from build123d import *

# Parameters (mm, degrees)
SKIZZE1_W                       = 26
SKIZZE1_H                       = 15
AUFSATZ_LINEAR_AUSTRAGEN1_DEPTH = 5
SCHNITT_LINEAR_AUSTRAGEN1_DEPTH = 15
SKIZZE3_W                       = 10
SKIZZE3_H                       = 15
SCHNITT_LINEAR_AUSTRAGEN2_DEPTH = 1.55


with BuildPart() as part:
    # Skizze1 → Aufsatz-Linear austragen1 (new body)
    with BuildSketch(Plane.XY):
        with Locations((13, 7.5)):
            Rectangle(SKIZZE1_W, SKIZZE1_H)
    extrude(amount=AUFSATZ_LINEAR_AUSTRAGEN1_DEPTH)

    # Skizze2 → Schnitt-Linear austragen1 (cut)
    with BuildSketch(Plane.ZY):
        with BuildLine():
            Line((5, 9.247140521), (5, 5.752859479))
            ThreePointArc((5, 5.752859479), (4.45, 7.5), (5, 9.247140521))
        make_face()
    extrude(amount=-SCHNITT_LINEAR_AUSTRAGEN1_DEPTH, mode=Mode.SUBTRACT)

    # Skizze3 → Schnitt-Linear austragen2 (cut)
    with BuildSketch(Plane.XY.offset(5)):
        with Locations((21, 7.5)):
            Rectangle(SKIZZE3_W, SKIZZE3_H)
    extrude(amount=-SCHNITT_LINEAR_AUSTRAGEN2_DEPTH, mode=Mode.SUBTRACT)


solid = part.part
Could you check a few things on this model? Use its own coordinates, in mm. A direction names the side the tool comes from. Round coordinates to 2 decimals unless told otherwise and drop trailing zeros. Loops run counter-clockwise (first coordinate to the right, second up) from the corner with the lowest first, then second, coordinate; pieces in that order, holes last. Notation, with made-up numbers: (56, 16.5) -> (100, 16.5) arc R13 ccw to (100, 26.5) -> close; hole circle Ø9 at (18, 13.5). An arc over 180 degrees is marked (long way). Use CSV: the item, a comma, the result in double quotes.
(1) Suppose I cut it at B-B on x = 13. Write out the boundary of the cut face in (y, z).
Return value:
outline,"(0, 0) -> (15, 0) -> (15, 5) -> (9.25, 5) arc R3.05 cw to (5.75, 5) -> (0, 5) -> close"
(2) Suppose I cut it at A-A on y = 7.5. Write out the boundary of the cut face in (x, z), plus the area to 3 significant figures.
Return value:
outline,"(0, 0) -> (26, 0) -> (26, 3.45) -> (16, 3.45) -> (16, 5) -> (15, 5) -> (15, 4.45) -> (0, 4.45) -> close"
area,"106 mm²"
(3) Suppose I cut it at C-C on z = 4. Write out the boundary of the cut face in (x, y), plus the area to 3 significant figures.
Return value:
outline,"(0, 0) -> (16, 0) -> (16, 15) -> (0, 15) -> close"
area,"240 mm²"
(4) Suppose I cut it at D-D on y = 2.75. Write out the boundary of the cut face in (x, z), plus the area to 4 significant figures.
Return value:
outline,"(0, 0) -> (26, 0) -> (26, 3.45) -> (16, 3.45) -> (16, 5) -> (0, 5) -> close"
area,"114.5 mm²"
(5) Will these pins go through, and if not, where does the flat tip stop? pin 1 Ø8 at (x, y) = (4, 3.5) entering from -Z; pin 2 Ø2 at (y, z) = (2, 4.5) entering from +X.
Return value:
pin 1,"stops at z = 0"
pin 2,"stops at x = 16"
(6) For faces 1 (the flat face through (26, 7, 2)), 2 (the flat face through (21, 8, 3.45)), 3 (the cylindrical face through (7.4, 7.47, 4.45)), which set-ups out of +Z, -Z, +X, -X, +Y, -Y let a thin tool reach every point of the face, with its end or its side?
Return value:
face 1,"+Z, -Z, +X, +Y, -Y"
face 2,"+Z, +X, +Y, -Y"
face 3,"+Z, -X"
(7) If I drill on probe 1 along Z at (x, y) = (21, 2.25); probe 2 along X at (y, z) = (14, 4.4); probe 3 along X at (y, z) = (7.5, 4.85), over which ranges is the centre line in solid material (lowest first)? Write a range as [from, to].
Return value:
probe 1,"z = [0, 3.45]"
probe 2,"x = [0, 16]"
probe 3,"x = [15, 16]"
